Build history of the part. All positions in model axes, mm. A direction names the side the tool comes from. Round coordinates to 2 decimals unless told otherwise and drop trailing zeros. Write each loop counter-clockwise with the first axis right and the second up, starting at its lowest first coordinate (ties: lowest second). Pieces come first, ordered by that corner, then holes.
1) Pull direction X, two halves, no side cores. Call faces 3 (the flat face through (6, 9.3, 6)), 4 (the cylindrical face through (-26.563, 7.55, -10.853)), 5 (the cylindrical face through (-4.769, 2.12, 21.477)), 6 (the cylindrical face through (-26.563, 7.55, 10.704)): +X half, -X half, draft (parallel to the pull), parting line (faces both ways), or undercut.
2) Wall check: probe 1 along Y at (x, z) = (6.5, -20.5); probe 2 along X at (y, z) = (8, 7); probe 3 along Z at (x, y) = (7, -1.25). Give the ranges that are in metal, low to high.
3) Which spindle directions (+Z, -Z, +X, -X, +Y, -Y) get a long thin tool onto all of the face, cutting with end or side? Do faces 1 (the cylindrical face through (-11.99, -4.07, 0.53)), 2 (the cylindrical face through (-0.369, 7.55, -25.897)). Say none if no direction does.
4) Saw through at B-B (y = -6.5). Write the cut outline in (x, z).
5) Saw through at D-D (x = 7). Write the cut outline in (y, z).
6) Flat gauge pins, fed straight in: pin 1 (1 mm diameter, centred on x = 2.5, y = 6.5, fed in from +Z); pin 2 (1.5 mm diameter, centred on x = -20.5, z = -16.5, fed in from -Y); pin 3 (2.5 mm diameter, centred on x = 0, z = 7, fed in from +Y); pin 4 (5 mm diameter, centred on x = 12, y = 3.5, fed in from +Z). Where does each tip first touch, or does it go through?
7) Saw through at A-A (y = 3.5). Write the cut outline in (x, z), plus the area to 3 significant figures.
8) Saw through at C-C (z = 0). State how many separate pieces and enclosed holes the cut face has, plus the area to 3 significant figures.
from build123d import *

# Parameters (mm, degrees)
SKETCH1_R                                       = 22
BOSS_EXTRUDE1_DEPTH                             = 4.3
SKETCH2_R                                       = 12
BOSS_EXTRUDE2_DEPTH                             = 8.25
SKETCH3_R                                       = 1.65
CUT_EXTRUDE2_DEPTH                              = 14.5
SKETCH4_R                                       = 30.87
SKETCH4_R_2                                     = 1.65
BOSS_EXTRUDE4_DEPTH                             = 5
SKETCH6_R                                       = 1.65
CUT_EXTRUDE4_DEPTH                              = 10
CSK_FOR_M3_FLAT_HEAD_MACHINE_SCREW2_D           = 3.4
CSK_FOR_M3_FLAT_HEAD_MACHINE_SCREW2_CSINK_D     = 6.3
CSK_FOR_M3_FLAT_HEAD_MACHINE_SCREW2_CSINK_ANGLE = 90
SKETCH5_R                                       = 1.65
CUT_EXTRUDE3_DEPTH                              = 25
CSK_FOR_M3_FLAT_HEAD_MACHINE_SCREW3_D           = 3.4
CSK_FOR_M3_FLAT_HEAD_MACHINE_SCREW3_CSINK_D     = 6.3
CSK_FOR_M3_FLAT_HEAD_MACHINE_SCREW3_CSINK_ANGLE = 90


with BuildPart() as part:
    # Sketch1 → Boss-Extrude1 (new body)
    with BuildSketch(Plane(origin=(0, 0, 0), x_dir=(1, 0, 0), z_dir=(0, 1, 0))):
        Circle(SKETCH1_R)
    extrude(amount=BOSS_EXTRUDE1_DEPTH)

    # Sketch2 → Boss-Extrude2 (add)
    with BuildSketch(Plane.XZ):
        Circle(SKETCH2_R)
    extrude(amount=BOSS_EXTRUDE2_DEPTH)

    # Sketch3 → Cut-Extrude2 (cut)
    with BuildSketch(Plane(origin=(0, 4.3, 0), x_dir=(1, 0, 0), z_dir=(0, 1, 0))):
        Circle(SKETCH3_R)
        with Locations((0, 7)):
            Circle(SKETCH3_R)
        with Locations((7, 0)):
            Circle(SKETCH3_R)
        with Locations((0, -7)):
            Circle(SKETCH3_R)
        with Locations((-7, 0)):
            Circle(SKETCH3_R)
    extrude(amount=-CUT_EXTRUDE2_DEPTH, mode=Mode.SUBTRACT)

    # Sketch4 → Boss-Extrude4 (add)
    with BuildSketch(Plane(origin=(0, 4.3, 0), x_dir=(1, 0, 0), z_dir=(0, 1, 0))):
        Circle(SKETCH4_R)
        Circle(SKETCH4_R_2, mode=Mode.SUBTRACT)
        with Locations((0, 7)):
            Circle(SKETCH4_R_2, mode=Mode.SUBTRACT)
        with Locations((7, 0)):
            Circle(SKETCH4_R_2, mode=Mode.SUBTRACT)
        with Locations((0, -7)):
            Circle(SKETCH4_R_2, mode=Mode.SUBTRACT)
        with Locations((-7, 0)):
            Circle(SKETCH4_R_2, mode=Mode.SUBTRACT)
        with Locations((0, -17)):
            Circle(SKETCH4_R_2, mode=Mode.SUBTRACT)
        with Locations((0, 17)):
            Circle(SKETCH4_R_2, mode=Mode.SUBTRACT)
    extrude(amount=BOSS_EXTRUDE4_DEPTH)

    # Sketch6 → Cut-Extrude4 (cut)
    with BuildSketch(Plane(origin=(0, 9.3, 0), x_dir=(1, 0, 0), z_dir=(0, 1, 0))):
        with Locations((0, 27.5567407)):
            Circle(SKETCH6_R)
        with Locations((0, -27.5567407)):
            Circle(SKETCH6_R)
        with Locations((-24.864837492, -10.77837035)):
            Circle(SKETCH6_R)
        with Locations((-24.864837492, 10.77837035)):
            Circle(SKETCH6_R)
        with Locations((-27.5567407, 0)):
            Circle(SKETCH6_R)
        with Locations((27.5567407, 0)):
            Circle(SKETCH6_R)
        with Locations((24.864837492, -10.77837035)):
            Circle(SKETCH6_R)
        with Locations((24.864837492, 10.77837035)):
            Circle(SKETCH6_R)
    extrude(amount=-CUT_EXTRUDE4_DEPTH, mode=Mode.SUBTRACT)

    # CSK for M3 Flat Head Machine Screw2 (through all)
    with Locations(Plane(origin=(0, 4.3, 0), x_dir=(-1, 0, 0), z_dir=(0, -1, 0))):
        with Locations((0, -27.5567407), (-24.864837492, -10.77837035), (-27.5567407, 0), (-24.864837492, 10.77837035), (0, 27.5567407), (24.864837492, 10.77837035), (27.5567407, 0), (24.864837492, -10.77837035)):
            CounterSinkHole(CSK_FOR_M3_FLAT_HEAD_MACHINE_SCREW2_D / 2, CSK_FOR_M3_FLAT_HEAD_MACHINE_SCREW2_CSINK_D / 2, counter_sink_angle=CSK_FOR_M3_FLAT_HEAD_MACHINE_SCREW2_CSINK_ANGLE)

    # Sketch5 → Cut-Extrude3 (cut)
    with BuildSketch(Plane(origin=(0, 9.3, 0), x_dir=(1, 0, 0), z_dir=(0, 1, 0))):
        with Locations((0, -7)):
            Circle(SKETCH5_R)
        with Locations((0, 7)):
            Circle(SKETCH5_R)
        with Locations((0, -17)):
            Circle(SKETCH5_R)
        with Locations((0, 17)):
            Circle(SKETCH5_R)
    extrude(amount=-CUT_EXTRUDE3_DEPTH, mode=Mode.SUBTRACT)

    # CSK for M3 Flat Head Machine Screw3 (through all)
    with Locations(Plane(origin=(0, 0, 0), x_dir=(-1, 0, 0), z_dir=(0, -1, 0))):
        with Locations((0, -17), (0, 17)):
            CounterSinkHole(CSK_FOR_M3_FLAT_HEAD_MACHINE_SCREW3_D / 2, CSK_FOR_M3_FLAT_HEAD_MACHINE_SCREW3_CSINK_D / 2, counter_sink_angle=CSK_FOR_M3_FLAT_HEAD_MACHINE_SCREW3_CSINK_ANGLE)


solid = part.part
Evaluation:
1. face 3: draft
1. face 4: undercut
1. face 5: parting line
1. face 6: undercut
2. probe 1: y = 0 to 9.3
2. probe 2: x = -30.07 to -1.65, 1.65 to 30.07
2. probe 3: z = -9.75 to -1.65, 1.65 to 9.75
3. face 1: -Y
3. face 2: +Y, -Y
4. outline: circle Ø24 at (0, 0); hole circle Ø3.3 at (-7, 0); hole circle Ø3.3 at (0, -7); hole circle Ø3.3 at (0, 0); hole circle Ø3.3 at (0, 7); hole circle Ø3.3 at (7, 0)
5. outline: (-8.25, -9.75) - (0, -9.75) - (0, -20.86) - (4.3, -20.86) - (4.3, -30.07) - (9.3, -30.07) - (9.3, -1.65) - (-8.25, -1.65) - close; (-8.25, 1.65) - (9.3, 1.65) - (9.3, 30.07) - (4.3, 30.07) - (4.3, 20.86) - (0, 20.86) - (0, 9.75) - (-8.25, 9.75) - close
6. pin 1: stops at z = 30.81
6. pin 2: stops at y = 4.3
6. pin 3: passes through
6. pin 4: stops at z = 29.33
7. outline: circle Ø44 at (0, 0); hole circle Ø3.3 at (-7, 0); hole circle Ø3.4 at (0, -17); hole circle Ø3.4 at (0, 17); hole circle Ø3.3 at (0, -7); hole circle Ø3.3 at (0, 0); hole circle Ø3.3 at (0, 7); hole circle Ø3.3 at (7, 0)
7. area: 1,460 mm2
8. separate pieces: 6
8. enclosed holes: 0
8. area: 484 mm2
